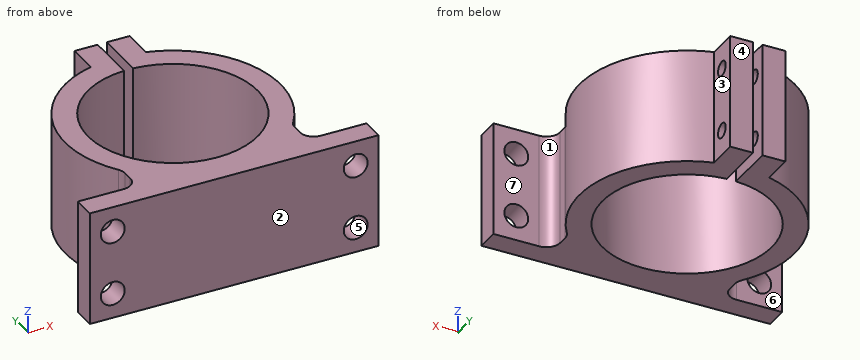
from build123d import *

# Parameters (mm, degrees)
BOSS_EXTRUDE1_DEPTH = 25
SKETCH2_W           = 25
SKETCH2_H           = 5
BOSS_EXTRUDE2_DEPTH = 13
FILLET1_R           = 3
SKETCH3_R           = 2.6
CUT_EXTRUDE1_DEPTH  = 65.222664554
FILLET2_R           = 3
SKETCH4_R           = 1.6
CUT_EXTRUDE2_DEPTH  = 54.850765737


with BuildPart() as part:
    # Sketch1 → Boss-Extrude1 (new body)
    with BuildSketch(Plane.XY):
        with BuildLine():
            Line((-18.5, -25.6), (18.5, -25.6))
            Line((18.5, -25.6), (18.5, -14.491376746))
            ThreePointArc((18.5, -14.491376746), (22.27678764, 7.482962811), (6, 22.721135535))
            Line((6, 22.721135535), (6, 29.472953202))
            Line((6, 29.472953202), (1, 29.472953202))
            Line((1, 29.472953202), (1, 18.472953202))
            ThreePointArc((1, 18.472953202), (0, -18.5), (-1, 18.472953202))
            Line((-1, 18.472953202), (-1, 29.472953202))
            Line((-1, 29.472953202), (-6, 29.472953202))
            Line((-6, 29.472953202), (-6, 22.721135535))
            ThreePointArc((-6, 22.721135535), (-22.27678764, 7.482962811), (-18.5, -14.491376746))
            Line((-18.5, -14.491376746), (-18.5, -25.6))
        make_face()
    extrude(amount=BOSS_EXTRUDE1_DEPTH)

    # Sketch2 → Boss-Extrude2 (add)
    with BuildSketch(Plane.ZY.offset(18.5)):
        with Locations((12.5, -23.1)):
            Rectangle(SKETCH2_W, SKETCH2_H)
    boss_extrude2 = extrude(amount=BOSS_EXTRUDE2_DEPTH)

    # Fillet1
    fillet1_edges = [part.edges().sort_by_distance(p)[0] for p in [
        (-18.5, -14.491376746, 12.5),
        (-18.5, -20.6, 12.5),
    ]]
    fillet(fillet1_edges, radius=FILLET1_R)

    # Sketch3 → Cut-Extrude1 (cut, through all)
    with BuildSketch(Plane(origin=(0, -20.6, 0), x_dir=(1, 0, 0), z_dir=(0, 1, 0))):
        with Locations(Location((-26.5, -19.5, 0), (0, 0, 270))):
            Circle(SKETCH3_R)
        with Locations(Location((-26.5, -5.5, 0), (0, 0, 270))):
            Circle(SKETCH3_R)
    cut_extrude1 = extrude(amount=-CUT_EXTRUDE1_DEPTH, mode=Mode.SUBTRACT)

    # Mirror3: Boss-Extrude2, Cut-Extrude1 across plane
    add(boss_extrude2.mirror(Plane(origin=(0, 0, 0), x_dir=(0, 0, 1), z_dir=(1, 0, 0))))
    add(cut_extrude1.mirror(Plane(origin=(0, 0, 0), x_dir=(0, 0, 1), z_dir=(1, 0, 0))), mode=Mode.SUBTRACT)

    # Fillet2
    fillet2_edges = [part.edges().sort_by_distance(p)[0] for p in [
        (18.5, -14.491376746, 12.5),
        (18.5, -20.6, 12.5),
    ]]
    fillet(fillet2_edges, radius=FILLET2_R)

    # Sketch4 → Cut-Extrude2 (cut, through all)
    with BuildSketch(Plane.ZY.offset(6)):
        with Locations(Location((19.5, 25.972953202, 0), (0, 0, 270))):
            Circle(SKETCH4_R)
        with Locations(Location((5.5, 25.972953202, 0), (0, 0, 270))):
            Circle(SKETCH4_R)
    extrude(amount=-CUT_EXTRUDE2_DEPTH, mode=Mode.SUBTRACT)


solid = part.part
Check sheet for the modelled part. Datum: model origin and axes. Units: mm. Face numbers are marked on the shaded views. A direction names the side the tool comes from. Give positions to 0.01 mm unless a question says otherwise; leave off trailing zeros. Order: outer loops, then holes, each group sorted by start corner. A loop starts at its lowest first (then second) coordinate and runs counter-clockwise, first axis right, second up. Notation, with made-up numbers: M -33.5,-36 L -5.5,-36 A21 ccw -5.5,-8 Z; hole C 55.25,-33 d2. An arc over 180 degrees is marked long. Answer as CSV lines item,"result". Start each with the question number.
Item 1: Cross-section at A-A on x = -26.5. Enter the section's corners in (y, z).
Item 2: Cross-section at C-C on z = 15.25. Enter the section's corners in (x, y), plus the area to 3 significant figures.
Item 3: Cross-section at B-B on y = 0. Enter the section's corners in (x, z), plus the area to 3 significant figures.
Item 4: Gauge pin test, flat ends, axial feed: P1, Ø9, axis at y = 23.5, z = 11, coming from the +X side; P2, Ø4, axis at y = -2, z = 11.5, coming from the +X side; P3, Ø5, axis at y = 25.97, z = 5.5, coming from the +X side. Record the tip position at first contact, or that the pin passes through.
Item 5: Tool access check on the marked faces 1, 2 and 3. Record the directions out of +Z, -Z, +X, -X, +Y, -Y that give a thin tool (end or side, any length) a straight path to the whole face; none if there is none.
Item 6: Thickness scan on line 1 (X direction, y = -24.35, z = 19.5); line 2 (Z direction, x = 26.5, y = -24); line 3 (X direction, y = 0, z = 6). Record the ranges inside material, lowest first. Write a range as [from, to].
Item 7: Cross-section at D-D on x = -7. Enter the section's corners in (y, z), plus the area to 3 significant figures.
Item 8: Mould release check, pull along Y, two halves, no side actions. Record for the marked faces 4, 5, 6 and 7: +Y half, -Y half, draft (parallel to the pull), parting line (faces both ways), or undercut.
Established:
1,outline,"M -25.6,0 L -20.6,0 L -20.6,2.9 L -25.6,2.9 Z; M -25.6,8.1 L -20.6,8.1 L -20.6,16.9 L -25.6,16.9 Z; M -25.6,22.1 L -20.6,22.1 L -20.6,25 L -25.6,25 Z"
2,outline,"M -31.5,-25.6 L 31.5,-25.6 L 31.5,-20.6 L 21.5,-20.6 A3 cw 18.5,-17.6 L 18.5,-15.49 A3 cw 19.07,-13.74 A23.5 ccw 6,22.72 L 6,29.47 L 1,29.47 L 1,18.47 A18.5 cw long -1,18.47 L -1,29.47 L -6,29.47 L -6,22.72 A23.5 ccw -19.07,-13.74 A3 cw -18.5,-15.49 L -18.5,-17.6 A3 cw -21.5,-20.6 L -31.5,-20.6 Z"
2,area,"1,030 mm^2"
3,outline,"M -23.5,0 L -18.5,0 L -18.5,25 L -23.5,25 Z; M 18.5,0 L 23.5,0 L 23.5,25 L 18.5,25 Z"
3,area,"250 mm^2"
4,P1,"stops at x = 13.83"
4,P2,"stops at x = 23.5"
4,P3,"stops at x = 6"
5,face 1,"+Z, -Z, +X"
5,face 2,"+Z, -Z, +X, -X, -Y"
5,face 3,"+Z, -Z, +X, +Y"
6,line 1,"x = [-31.5, -29.1], [-23.9, 23.9], [29.1, 31.5]"
6,line 2,"z = [0, 2.9], [8.1, 16.9], [22.1, 25]"
6,line 3,"x = [-23.5, -18.5], [18.5, 23.5]"
7,outline,"M -25.6,0 L -17.12,0 L -17.12,25 L -25.6,25 Z; M 17.12,0 L 22.43,0 L 22.43,25 L 17.12,25 Z"
7,area,"345 mm^2"
8,face 4,"+Y half"
8,face 5,"draft"
8,face 6,"undercut"
8,face 7,"undercut"
